Could you check a few things on this drawing? It's one solid part, dimensions in mm from its lowest x, y, z. Give positions to 0.01 mm unless a question says otherwise; leave off trailing zeros. Loops run counter-clockwise (first coordinate to the right, second up) from the corner with the lowest first, then second, coordinate; pieces in that order, holes last. Notation, with made-up numbers: M 84,-40 L 93,-40 A21 ccw 93,-24 Z; hole C 33.5,48 d2. An arc over 180 degrees is marked long. Return JSON: item names as keys, results as strings. Group by question number.
1. Please list where these lines run through material, in increasing order: line 1 (Z direction, x = 12.7, y = 4.5); line 2 (Y direction, x = 12.7, z = 2); line 3 (Z direction, x = 12.7, y = 5.25).
2. If we section it at B-B (z = 12.7): Write out the boundary of the cut face in (x, y).
3. If we mould it in two halves opening along X, with no side actions, what happens to the marked faces 1, 2 and 3? For each: +X half, -X half, draft (parallel to the pull), parting line (faces both ways), or undercut.
4. If we section it at A-A (x = 12.7): Write out the boundary of the cut face in (y, z).
5. If we section it at C-C (y = 2.5): Write out the boundary of the cut face in (x, z), plus the area to 3 significant figures.
6. If we section it at D-D (x = 9): Write out the boundary of the cut face in (y, z) (1 decimal).
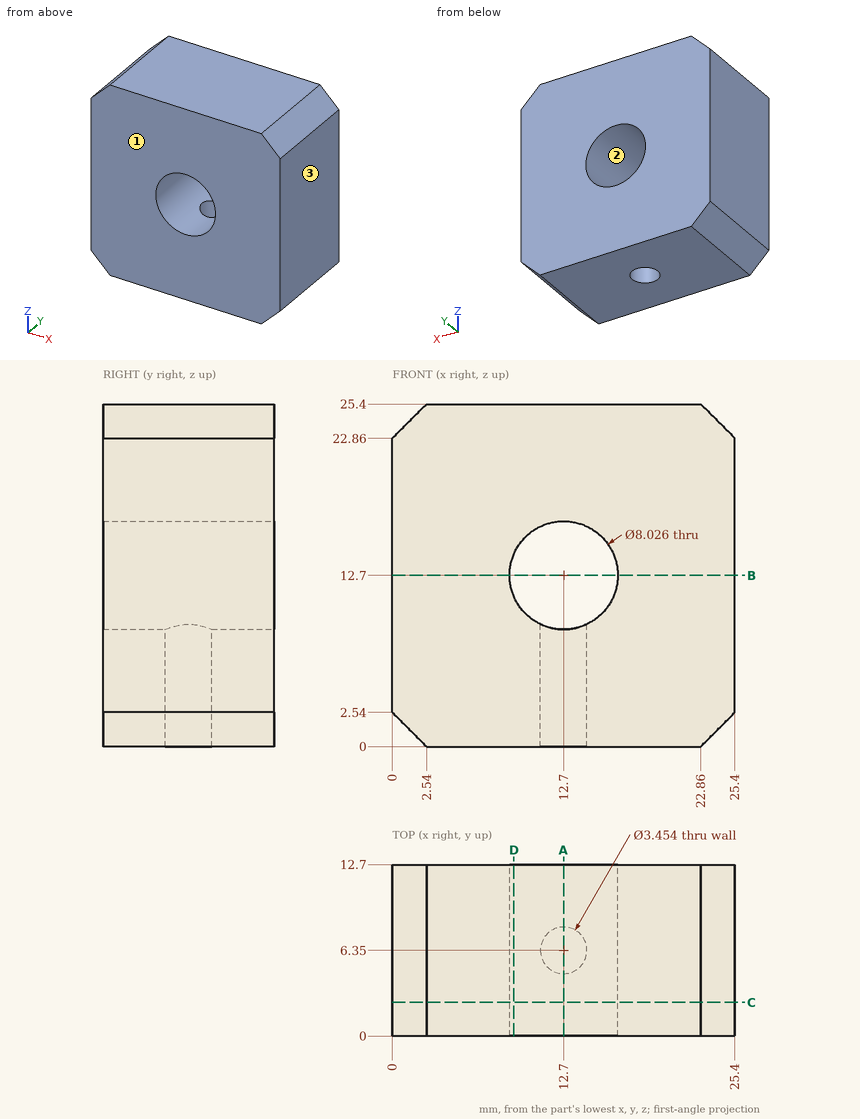
Answer:
{
 "1": {"line 1": "z = 0 to 8.69, 16.71 to 25.4", "line 2": "y = 0 to 4.62, 8.08 to 12.7", "line 3": "z = 16.71 to 25.4"},
 "2": {"outline": "M 0,0 L 8.69,0 L 8.69,12.7 L 0,12.7 Z; M 16.71,0 L 25.4,0 L 25.4,12.7 L 16.71,12.7 Z"},
 "3": {"face 1": "draft", "face 2": "undercut", "face 3": "+X half"},
 "4": {"outline": "M 0,0 L 4.62,0 L 4.62,8.69 L 0,8.69 Z; M 0,16.71 L 12.7,16.71 L 12.7,25.4 L 0,25.4 Z; M 8.08,0 L 12.7,0 L 12.7,8.69 L 8.08,8.69 Z"},
 "5": {"outline": "M 0,2.54 L 2.54,0 L 22.86,0 L 25.4,2.54 L 25.4,22.86 L 22.86,25.4 L 2.54,25.4 L 0,22.86 Z; hole C 12.7,12.7 d8.03", "area": "582 mm²"},
 "6": {"outline": "M 0,0 L 12.7,0 L 12.7,11.1 L 0,11.1 Z; M 0,14.3 L 12.7,14.3 L 12.7,25.4 L 0,25.4 Z"}
}
